Here's how the part is built. I have some questions about the finished solid (model axes, mm). A direction names the side the tool comes from. Give positions to 0.01 mm unless a question says otherwise; leave off trailing zeros. Loops run counter-clockwise (first coordinate to the right, second up) from the corner with the lowest first, then second, coordinate; pieces in that order, holes last.
Q1. I'm going to push flat-ended pins straight in: P1, Ø2.5, axis at y = 14, z = 2, coming from the -X side; P2, Ø1.5, axis at y = -7.5, z = 2, coming from the +X side; P3, Ø1.5, axis at x = -32.5, z = 3.5, coming from the -Y side. Where does each tip first touch, or does it pass through?
Q2. Suppose I cut it at C-C (x = -9). List the corners of the cut face in (y, z) for me, and give its area (3 significant figures).
Q3. I need wall thicknesses on probe 1 along X at (y, z) = (-13, 3.85); probe 2 along Y at (x, z) = (9, 2.4); probe 3 along Y at (x, z) = (-11, 3.85). Which ranges of each line are inside material? Lowest first, please.
Q4. Suppose I cut it at A-A (y = 14). List the corners of the cut face in (x, z) for me, and give its area (3 significant figures).
Q5. Thinking about a two-plate mould opening in Y: for faces 1 (the face through (0, 8, 0)), 2 (the face through (-32, 5.5, 2)), 3 (the face through (0, -5, 2)), which applies, pulls with the +Y half, pulls with the -Y half, needs draft (parallel to the pull), parting line crosses it, or undercut?
Q6. Suppose I cut it at D-D (y = 10). List the corners of the cut face in (x, z) for me, and give its area (3 significant figures).
Q7. For faces 4 (the face through (10, -15, 2)), 5 (the face through (32, -5.5, 2)), 6 (the face through (-30, -9, 2)), 7 (the face through (30, 9, 2)), 8 (the face through (10, 15, 2)), which set-ups out of +Z, -Z, +X, -X, +Y, -Y let a thin tool reach every point of the face, with its end or its side?
```python
from build123d import *

# Parameters (mm, degrees)
SKETCH1_W           = 40
SKETCH1_H           = 10
BOSS_EXTRUDE1_DEPTH = 5


with BuildPart() as part:
    # Sketch1 → Boss-Extrude1 (new body)
    with BuildSketch(Plane.XY):
        Polygon((-30, -12.5), (-20, -12.5), (-20, -17.5), (-10, -17.5), (-10, -12.5), (10, -12.5), (10, -17.5), (20, -17.5), (20, -12.5), (30, -12.5), (30, -5.5), (35, -5.5), (35, 5.5), (30, 5.5), (30, 12.5), (20, 12.5), (20, 17.5), (10, 17.5), (10, 12.5), (-10, 12.5), (-10, 17.5), (-20, 17.5), (-20, 12.5), (-30, 12.5), (-30, 5.5), (-35, 5.5), (-35, -5.5), (-30, -5.5), align=None)
        Rectangle(SKETCH1_W, SKETCH1_H, mode=Mode.SUBTRACT)
    extrude(amount=BOSS_EXTRUDE1_DEPTH)


solid = part.part
```
Solutions:
1. P1: stops at x = -20
1. P2: stops at x = 30
1. P3: stops at y = -5.5
2. outline: (-12.5, 0) - (-5, 0) - (-5, 5) - (-12.5, 5) - close; (5, 0) - (12.5, 0) - (12.5, 5) - (5, 5) - close
2. area: 75.0 mm2
3. probe 1: x = -20 to -10, 10 to 20
3. probe 2: y = -12.5 to -5, 5 to 12.5
3. probe 3: y = -17.5 to -5, 5 to 17.5
4. outline: (-20, 0) - (-10, 0) - (-10, 5) - (-20, 5) - close; (10, 0) - (20, 0) - (20, 5) - (10, 5) - close
4. area: 100 mm2
5. face 1: needs draft
5. face 2: pulls with the +Y half
5. face 3: undercut
6. outline: (-30, 0) - (30, 0) - (30, 5) - (-30, 5) - close
6. area: 300 mm2
7. face 4: +Z, -Z, -Y
7. face 5: +Z, -Z, +X, -Y
7. face 6: +Z, -Z, -X, -Y
7. face 7: +Z, -Z, +X, +Y
7. face 8: +Z, -Z, +Y
